```python
from build123d import *

# Parameters (mm, degrees)
BOSS_EXTRUDE1_DEPTH = 3
SKETCH2_W           = 57.45
SKETCH2_H           = 28.45
BOSS_EXTRUDE2_DEPTH = 1.7
SKETCH3_R           = 1.45
CUT_EXTRUDE1_DEPTH  = 5.7
CUT_EXTRUDE2_DEPTH  = 2


with BuildPart() as part:
    # Sketch1 → Boss-Extrude1 (new body)
    with BuildSketch(Plane(origin=(0, 0, 0), x_dir=(1, 0, 0), z_dir=(0, 1, 0))):
        with BuildLine():
            Line((-32.939945355, 17.5), (-32.939945355, -17.5))
            ThreePointArc((-32.939945355, -17.5), (37.3, 0), (-32.939945355, 17.5))
        make_face()
    extrude(amount=BOSS_EXTRUDE1_DEPTH)

    # Sketch2 → Boss-Extrude2 (add)
    with BuildSketch(Plane(origin=(0, 3, 0), x_dir=(1, 0, 0), z_dir=(0, 1, 0))):
        with BuildLine():
            Line((-32.939945355, 17.5), (-32.939945355, -17.5))
            ThreePointArc((-32.939945355, -17.5), (37.3, 0), (-32.939945355, 17.5))
        make_face()
        with Locations((-2.714945355, 0)):
            Rectangle(SKETCH2_W, SKETCH2_H, mode=Mode.SUBTRACT)
    extrude(amount=BOSS_EXTRUDE2_DEPTH)

    # Sketch3 → Cut-Extrude1 (cut, through all)
    with BuildSketch(Plane(origin=(0, 4.7, 0), x_dir=(1, 0, 0), z_dir=(0, 1, 0))):
        with Locations((0, 15.5)):
            Circle(SKETCH3_R)
    cut_extrude1 = extrude(amount=-CUT_EXTRUDE1_DEPTH, mode=Mode.SUBTRACT)

    # Sketch4 → Cut-Extrude2 (cut)
    with BuildSketch(Plane.XZ):
        Polygon((2.886751346, -15.5), (1.443375673, -13), (-1.443375673, -13), (-2.886751346, -15.5), (-1.443375673, -18), (1.443375673, -18), align=None)
    cut_extrude2 = extrude(amount=-CUT_EXTRUDE2_DEPTH, mode=Mode.SUBTRACT)

    # Mirror2: Cut-Extrude1, Cut-Extrude2 across plane
    add(cut_extrude1.mirror(Plane.XY), mode=Mode.SUBTRACT)
    add(cut_extrude2.mirror(Plane.XY), mode=Mode.SUBTRACT)


solid = part.part
```
Here's how the part is built. I have some questions about the finished solid (model axes, mm). A direction names the side the tool comes from. Round coordinates to 2 decimals unless told otherwise and drop trailing zeros. Order: outer loops, then holes, each group sorted by start corner. A loop starts at its lowest first (then second) coordinate and runs counter-clockwise, first axis right, second up. Notation, with made-up numbers: M 16.5,-35 L 21.5,-35 A32 cw 21.5,-2 Z; hole C 73,-17.75 d10. An arc over 180 degrees is marked long. One line per question, with ' | ' between items.
1) I want a section at C-C, the plane z = 0. Write out the boundary of the cut face in (x, y), then the cut area to 3 significant figures.
Working result:
outline: M -32.94,0 L 37.3,0 L 37.3,4.7 L 26.01,4.7 L 26.01,3 L -31.44,3 L -31.44,4.7 L -32.94,4.7 Z | area: 232 mm²
2) If we mould it in two halves opening along X, with no side actions, what happens to faces 4 (the face through (-3, 3, 0)), 5 (the face through (26.01, 4, 0)), 6 (the face through (2, 4.7, 16))? For each: +X half, -X half, draft (parallel to the pull), parting line (faces both ways), or undercut.
Working result:
face 4: undercut | face 5: undercut | face 6: draft
3) I want a section at D-D, the plane z = 30. Write out the boundary of the cut face in (x, y), then the cut area to 3 significant figures.
Working result:
outline: M -22.17,0 L 22.17,0 L 22.17,4.7 L -22.17,4.7 Z | area: 208 mm²
4) I want a section at A-A, the plane y = 0.8. Write out the boundary of the cut face in (x, z), then the cut area to 3 significant figures.
Working result:
outline: M -32.94,-17.5 A37.3 ccw long -32.94,17.5 Z; hole M -2.89,-15.5 L -1.44,-18 L 1.44,-18 L 2.89,-15.5 L 1.44,-13 L -1.44,-13 Z; hole M -2.89,15.5 L -1.44,13 L 1.44,13 L 2.89,15.5 L 1.44,18 L -1.44,18 Z | area: 4,220 mm²
5) For pin 1 Ø0.6 at (x, y) = (0.5, 1.5) entering from +Z; pin 2 Ø0.8 at (x, y) = (-21, 3.5) entering from -Z; pin 3 Ø1.5 at (y, z) = (3, 20) entering from +X, each with a flat end and sliding along its axis, tell me the tip position at first contact or that it passes through.
Working result:
pin 1: z = 37.3 | pin 2: z = -31.1 | pin 3: x = 31.95
6) I need wall thicknesses on line 1 along Z through (x, y) = (0, 3.55); line 2 along Y through (x, z) = (25, 6.5); line 3 along Z through (x, y) = (-17, 4.25) (3 decimals). Which ranges of each line are inside material? Lowest first, please.
Working result:
line 1: -37.3 to -16.95, 16.95 to 37.3 | line 2: 0 to 3 | line 3: -33.201 to -14.225, 14.225 to 33.201
7) I want a section at B-B, the plane x = 8.5. Write out the boundary of the cut face in (y, z) (3 decimals).
Working result:
outline: M 0,-36.319 L 4.7,-36.319 L 4.7,-14.225 L 3,-14.225 L 3,14.225 L 4.7,14.225 L 4.7,36.319 L 0,36.319 Z
8) For faces 1 (the face through (2, 0, -1)), 2 (the face through (-2.155, 0.986, 14.232)), 3 (the face through (13, 4, -14.225)), which set-ups out of +Z, -Z, +X, -X, +Y, -Y let a thin tool reach every point of the face, with its end or its side?
Working result:
face 1: +Z, -Z, +X, -X, -Y | face 2: -Y | face 3: +Y
